Can you work these out from the model? Positions are in its coordinate system, mm. A direction names the side the tool comes from. Coordinates: 2 decimals unless noted, no trailing zeros. Order: outer loops, then holes, each group sorted by start corner. A loop starts at its lowest first (then second) coordinate and runs counter-clockwise, first axis right, second up. Notation, with made-up numbers: (-29, 18) -> (30, 18) arc R35 cw to (30, 53) -> close; hole circle Ø5 at (88, 31.25). An arc over 180 degrees is marked (long way). Return JSON: item names as keys, results as strings. Group by question number.
1) For faces 1 (the flat face through (-13, 41, 444)), 2 (the flat face through (-35, 68, 444)), 3 (the flat face through (20, 3, 444)), 4 (the flat face through (-15, 68, 444)), which set-ups out of +Z, -Z, +X, -X, +Y, -Y let a thin tool reach every point of the face, with its end or its side?
2) For pin 1 (4 mm diameter, centred on x = -3.5, y = 45.5, fed in from -Z); pin 2 (3 mm diameter, centred on y = 24.5, z = 497, fed in from -X); pin 3 (5 mm diameter, centred on x = 5, z = 774, fed in from +Y); pin 4 (11 mm diameter, centred on x = -28.5, z = 529.5, fed in from -Y), each with a flat end and sliding along its axis, tell me the tip position at first contact or that it passes through.
3) If we section it at C-C, the plane z = 310: Please give me the cut outline in (x, y).
4) If we section it at A-A, the plane y = 20.5: Please give me the cut outline in (x, z).
5) Thinking about a two-plate mould opening in X: for faces 5 (the flat face through (0, 44, 900)), 6 (the flat face through (40, 30, 444)), 7 (the flat face through (37, 30, 444)), which applies, +X half, -X half, draft (parallel to the pull), parting line (faces both ways), or undercut?
6) If we section it at B-B, the plane x = 25: Please give me the cut outline in (y, z).
7) If I drill on probe 1 along X at (y, z) = (40, 731.5); probe 2 along Y at (x, z) = (17, 615); probe 3 along X at (y, z) = (11.5, 853), over which ranges is the centre line in solid material (lowest first)? Write a range as from..to.
from build123d import *

# Parameters (mm, degrees)
SKETCH_W  = 34
SKETCH_H  = 54
PAD_DEPTH = 900


with BuildPart() as part:
    # Sketch → Pad (new body)
    with BuildSketch(Plane.XY):
        with BuildLine():
            Line((0, 0), (40, 0))
            Line((40, 0), (40, 60))
            Line((40, 60), (-15, 60))
            Line((-15, 75.5), (-15, 60))
            Line((-35, 75.5), (-15, 75.5))
            Line((-35, 60), (-35, 75.5))
            Line((-35, 60), (-40, 60))
            Line((-40, 60), (-40, 57))
            Line((-40, 57), (-18, 57))
            ThreePointArc((-13, 52), (-14.464466, 55.535534), (-18, 57))
            Line((-13, 52), (-13, 30))
            Line((-13, 30), (0, 30))
            Line((0, 30), (0, 0))
        make_face()
        with Locations((20, 30)):
            Rectangle(SKETCH_W, SKETCH_H, mode=Mode.SUBTRACT)
    extrude(amount=PAD_DEPTH)


solid = part.part
Result sheet:
{
 "1": {"face 1": "+Z, -Z, -X, -Y", "face 2": "+Z, -Z, -X, +Y", "face 3": "+Z, -Z", "face 4": "+Z, -Z, +X, +Y"},
 "2": {"pin 1": "stops at z = 0", "pin 2": "stops at x = 0", "pin 3": "stops at y = 60", "pin 4": "stops at y = 57"},
 "3": {"outline": "(-40, 57) -> (-18, 57) arc R5 cw to (-13, 52) -> (-13, 30) -> (0, 30) -> (0, 0) -> (40, 0) -> (40, 60) -> (-15, 60) -> (-15, 75.5) -> (-35, 75.5) -> (-35, 60) -> (-40, 60) -> close; hole (3, 3) -> (37, 3) -> (37, 57) -> (3, 57) -> close"},
 "4": {"outline": "(0, 0) -> (3, 0) -> (3, 900) -> (0, 900) -> close; (37, 0) -> (40, 0) -> (40, 900) -> (37, 900) -> close"},
 "5": {"face 5": "draft", "face 6": "+X half", "face 7": "undercut"},
 "6": {"outline": "(0, 0) -> (3, 0) -> (3, 900) -> (0, 900) -> close; (57, 0) -> (60, 0) -> (60, 900) -> (57, 900) -> close"},
 "7": {"probe 1": "x = -13..3, 37..40", "probe 2": "y = 0..3, 57..60", "probe 3": "x = 0..3, 37..40"}
}
